```python
from build123d import *
from build123d.topology import SkipClean

# Parameters (mm, degrees)
BOSS_EXTRU_1_DEPTH      = 3
BOSS_EXTRU_1_DEPTH_BACK = 3
ESQUISSE1_R             = 1.55
SKETCH1_W               = 14
SKETCH1_H               = 21
BOSS_EXTRUDE1_DEPTH     = 2
SKETCH3_R               = 1.55
CUT_EXTRUDE1_DEPTH      = 2
FILLET1_R               = 2
BOSS_EXTRUDE3_START     = -5
SKETCH4_R               = 5
SKETCH4_R_2             = 1.55
BOSS_EXTRUDE3_DEPTH     = 5


with BuildPart() as part:
    # Esquisse1 → Boss.-Extru.1 (new, two sides: drawn at the far end of the back side and taken through both)
    with BuildSketch(Plane.XY.offset(-BOSS_EXTRU_1_DEPTH_BACK)):
        with BuildLine():
            Line((-0.279242011, 4.9921963), (7.720757989, 4.9921963))
            Line((7.720757989, 4.9921963), (7.720757989, -4.9921963))
            Line((7.720757989, -4.9921963), (-0.279242011, -4.9921963))
            ThreePointArc((-0.279242011, -4.9921963), (-5, 0), (-0.279242011, 4.9921963))
        make_face()
        Circle(ESQUISSE1_R, mode=Mode.SUBTRACT)
    extrude(amount=BOSS_EXTRU_1_DEPTH + BOSS_EXTRU_1_DEPTH_BACK)

    # Sketch1 → Boss-Extrude1 (add)
    with BuildSketch(Plane(origin=(7.720757989, 0, 0), x_dir=(0, 0, -1), z_dir=(1, 0, 0))):
        Rectangle(SKETCH1_W, SKETCH1_H)
    extrude(amount=BOSS_EXTRUDE1_DEPTH)

    # Sketch3 → Cut-Extrude1 (cut)
    with BuildSketch(Plane.ZY.offset(-7.720757989)):
        with Locations((0, 7.5)):
            Circle(SKETCH3_R)
        with Locations((0, -7.5)):
            Circle(SKETCH3_R)
    extrude(amount=-CUT_EXTRUDE1_DEPTH, mode=Mode.SUBTRACT)

    # Fillet1
    fillet1_edges = [part.edges().sort_by_distance(p)[0] for p in [
        (8.720757989, -10.5, -7),
        (8.720757989, 10.5, -7),
        (8.720757989, 10.5, 7),
        (8.720757989, -10.5, 7),
    ]]
    fillet(fillet1_edges, radius=FILLET1_R)

    # Sketch4 → Boss-Extrude3 (add)
    with SkipClean():  # the faces are left unmerged after this step: merging them gives an invalid solid
        with BuildSketch(Plane.XY.offset(-3).offset(BOSS_EXTRUDE3_START)):
            Circle(SKETCH4_R)
            Circle(SKETCH4_R_2, mode=Mode.SUBTRACT)
        extrude(amount=BOSS_EXTRUDE3_DEPTH)


solid = part.part
```
For this review, take the finished solid that the model builds, in its own axes (mm). A direction names the side the tool comes from. Coordinates: 2 decimals unless noted, no trailing zeros. Write each loop counter-clockwise with the first axis right and the second up, starting at its lowest first coordinate (ties: lowest second). Pieces come first, ordered by that corner, then holes.
(1) Tool access review of faces 1 (the face through (6, 0, -3)), 2 (the face through (4, -4.992, 0)), 3 (the face through (3, 0, 3)), 4 (the face through (9, 0, -7)): name each direction out of +Z, -Z, +X, -X, +Y, -Y from which nothing blocks a thin tool from reaching the whole face with its end or side.
(2) Add section A-A on z = 0. Give the boundary of the cut face in (x, y), then the cut area to 3 significant figures.
(3) Add section D-D on z = -2.25. Give the boundary of the cut face in (x, y).
(4) Wall thickness on probe 1 along Y at (x, z) = (0, -5.5); probe 2 along Z at (x, y) = (0.75, 3.75); probe 3 along Y at (x, z) = (8.5, 1): over which ranges is each line inside the solid? List them lowest first.
(5) For pin 1 Ø3.5 at (y, z) = (7.5, 0) entering from -X; pin 2 Ø8 at (x, y) = (0, -1) entering from +Z; pin 3 Ø1.5 at (y, z) = (-6.5, 0) entering from +X; pin 4 Ø3 at (x, z) = (5.5, -1) entering from +Y, all flat-tipped, find the tip position at first contact; note any pin that passes through.
(6) Add section C-C on y = -7.5. Give the boundary of the cut face in (x, z).
(7) The part is to be moulded in two halves that separate along Y. For faces 5 (the face through (0.715, -1.375, -2.577)), 6 (the face through (8.73, -9.9, 6.43)), 7 (the face through (7.721, 0.1, 3.2)), say which applies: +Y half, -Y half, draft (parallel to the pull), parting line (faces both ways), or undercut.
Answer sheet:
1. face 1: -Z
1. face 2: +Z, -Z, -X, -Y
1. face 3: +Z, -X, +Y, -Y
1. face 4: -Z, +X, +Y, -Y
2. outline: (-0.28, -4.99) - (7.72, -4.99) - (7.72, -5.95) - (9.72, -5.95) - (9.72, 5.95) - (7.72, 5.95) - (7.72, 4.99) - (-0.28, 4.99) arc R5 ccw to start; (7.72, -10.5) - (9.72, -10.5) - (9.72, -9.05) - (7.72, -9.05) - close; (7.72, 9.05) - (9.72, 9.05) - (9.72, 10.5) - (7.72, 10.5) - close; hole circle Ø3.1 at (0, 0)
2. area: 138 mm2
3. outline: (-0.28, -4.99) - (7.72, -4.99) - (7.72, -10.5) - (9.72, -10.5) - (9.72, 10.5) - (7.72, 10.5) - (7.72, 4.99) - (-0.28, 4.99) arc R5 ccw to start; hole circle Ø3.1 at (0, 0)
4. probe 1: y = -5 to -1.55, 1.55 to 5
4. probe 2: z = -8 to 3
4. probe 3: y = -10.5 to -8.68, -6.32 to 6.32, 8.68 to 10.5
5. pin 1: stops at x = 7.72
5. pin 2: stops at z = 3
5. pin 3: stops at x = 9.72
5. pin 4: stops at y = 4.99
6. outline: (7.72, -7) - (9.72, -7) - (9.72, -1.55) - (7.72, -1.55) - close; (7.72, 1.55) - (9.72, 1.55) - (9.72, 7) - (7.72, 7) - close
7. face 5: undercut
7. face 6: -Y half
7. face 7: draft
